The listing builds one solid part. Answer for the finished solid, in the listing's coordinates (mm). Give positions to 0.01 mm unless a question says otherwise; leave off trailing zeros. Write each loop counter-clockwise with the first axis right and the second up, starting at its lowest first coordinate (ties: lowest second). Pieces come first, ordered by that corner, then holes. Notation, with made-up numbers: M -39,58 L 3,58 A19 ccw 3,84 Z; hole C -11.75,67.5 d1. An arc over 180 degrees is marked long. Answer as a JSON object with one key per item and string values.
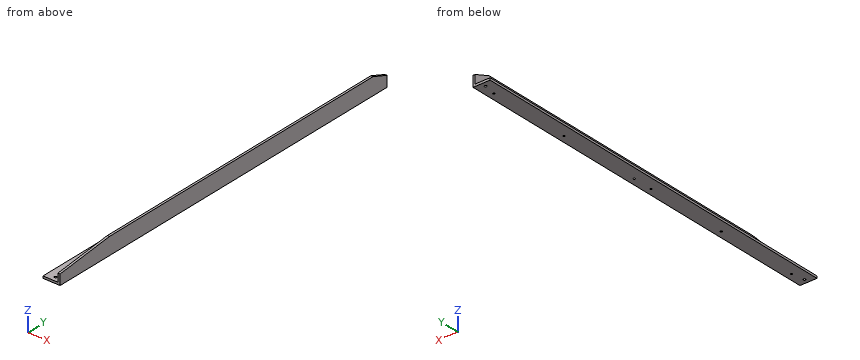
```python
from build123d import *

# Parameters (mm, degrees)
F1_DEPTH = 291
F4_SIZE2 = 25
F4_SIZE  = 9.5
F5_SIZE2 = 10.1
F5_SIZE  = 88
F7_R     = 1.75
F8_DEPTH = 3.2
F3_R     = 1.35
F9_DEPTH = 25


with BuildPart() as f1:
    # F0 (on Front) → F1 (new body, symmetric)
    with BuildSketch(Plane.XZ):
        Polygon((25.4, 12.7), (22.2, 12.7), (22.2, -9.5), (0, -9.5), (0, -12.7), (25.4, -12.7), align=None)
    extrude(amount=F1_DEPTH, both=True)

    # F4
    f4_edges = [f1.edges().sort_by_distance(p)[0] for p in [
        (23.8, 291, 12.7),
    ]]
    f4_side = f1.faces().sort_by_distance((23.8, 291, 12.34079))[0]
    chamfer(f4_edges, length=F4_SIZE, length2=F4_SIZE2, reference=f4_side)

    # F5
    f5_edges = [f1.edges().sort_by_distance(p)[0] for p in [
        (23.8, -291, 12.7),
    ]]
    f5_side = f1.faces().sort_by_distance((23.8, -12.5, 12.7))[0]
    chamfer(f5_edges, length=F5_SIZE, length2=F5_SIZE2, reference=f5_side)

    # F7 (on face) → F8 (cut, through all)
    with BuildSketch(Plane.XY.offset(-9.5)):
        with Locations((12.7, -283.8)):
            Circle(F7_R)
        with Locations((12.7, 283.8)):
            Circle(F7_R)
    extrude(amount=-F8_DEPTH, mode=Mode.SUBTRACT)

    # F3 (on face) → F9 (cut)
    with BuildSketch(Plane(origin=(0, 0, -12.7), x_dir=(1, 0, 0), z_dir=(0, 0, -1))):
        with Locations((16.2, 15)):
            Circle(F3_R)
        with Locations((16.2, -15)):
            Circle(F3_R)
        with Locations((16.2, 140)):
            Circle(F3_R)
        with Locations((16.2, 265)):
            Circle(F3_R)
        with Locations((16.2, -140)):
            Circle(F3_R)
        with Locations((16.2, -265)):
            Circle(F3_R)
    extrude(amount=-F9_DEPTH, mode=Mode.SUBTRACT)


solid = f1.part
```
1. A cutting plane is placed at A-A, the plane y = -43. Give the vertices of the cut face in (x, z), plus the area to 3 significant figures.
Verdict:
{"outline": "M 0,-12.7 L 25.4,-12.7 L 25.4,12.7 L 22.2,12.7 L 22.2,-9.5 L 0,-9.5 Z", "area": "152 mm2"}
2. Flat-ended cylindrical pins translate along their axes: pin 1 (3 mm diameter, centred on x = 16.2, y = 265, fed in from +Z); pin 2 (1.5 mm diameter, centred on y = 196.5, z = -4, fed in from -X). Find the tip coordinate at first contact, or state that the pin passes through.
Verdict:
{"pin 1": "stops at z = -9.5", "pin 2": "stops at x = 22.2"}
3. Consider line 1 along Y through (x, z) = (12.7, -11.5); line 2 along X through (y, z) = (283.8, -10.95); line 3 along X through (y, z) = (140.5, 8.5). Determine where each line is inside the solid, lowest interval first.
Verdict:
{"line 1": "y = -291 to -285.55, -282.05 to 282.05, 285.55 to 291", "line 2": "x = 0 to 10.95, 14.45 to 25.4", "line 3": "x = 22.2 to 25.4"}
4. A cutting plane is placed at B-B, the plane z = -3. Give the vertices of the cut face in (x, y).
Verdict:
{"outline": "M 22.2,-291 L 25.4,-291 L 25.4,291 L 22.2,291 Z"}
